```python
from build123d import *

# Parameters (mm, degrees)
SKETCH_1_R          = 20
EXTRUDE_1_DEPTH     = 200
SKETCH_2_W          = 40
SKETCH_2_H          = 40
EXTRUDE_2_DEPTH     = 50
SKETCH_3_W          = 100
SKETCH_3_H          = 30
EXTRUDE_3_DEPTH     = 40
SKETCH_4_W          = 100
SKETCH_4_H          = 30
EXTRUDE_4_DEPTH     = 40
FILLET_1_R          = 10
SKETCH_10_R         = 10
CUT_EXTRUDE_1_DEPTH = 20
EXTRUDE_6_DEPTH     = 20
EXTRUDE_7_DEPTH     = 20


with BuildPart() as part:
    # 스케치1 → 보스-돌출1 (new body)
    with BuildSketch(Plane.XY):
        Circle(SKETCH_1_R)
    extrude(amount=EXTRUDE_1_DEPTH)

    # 스케치2 → 보스-돌출2 (add)
    with BuildSketch(Plane(origin=(0, 0, 0), x_dir=(0, 0, -1), z_dir=(1, 0, 0))):
        with Locations((-20, 0)):
            Rectangle(SKETCH_2_W, SKETCH_2_H)
        with Locations((-120, 0)):
            Rectangle(SKETCH_2_W, SKETCH_2_H)
    extrude(amount=EXTRUDE_2_DEPTH)

    # 스케치3 → 보스-돌출3 (add)
    with BuildSketch(Plane(origin=(0, 0, 0), x_dir=(-1, 0, 0), z_dir=(0, 0, -1))):
        with Locations((-100, -31)):
            Rectangle(SKETCH_3_W, SKETCH_3_H)
        with Locations((-100, 31)):
            Rectangle(SKETCH_3_W, SKETCH_3_H)
    extrude(amount=-EXTRUDE_3_DEPTH)

    # 스케치4 → 보스-돌출4 (add)
    with BuildSketch(Plane(origin=(0, 0, 100), x_dir=(-1, 0, 0), z_dir=(0, 0, -1))):
        with Locations((-100, -31)):
            Rectangle(SKETCH_4_W, SKETCH_4_H)
        with Locations((-100, 31)):
            Rectangle(SKETCH_4_W, SKETCH_4_H)
    extrude(amount=-EXTRUDE_4_DEPTH)

    # 필렛1
    fillet_1_edges = [part.edges().sort_by_distance(p)[0] for p in [
        (50, -20, 20),
        (50, 20, 120),
        (50, -20, 120),
        (50, -16, 20),
        (50, 16, 20),
        (50, -16, 120),
        (50, 16, 120),
        (50, 20, 20),
    ]]
    fillet(fillet_1_edges, radius=FILLET_1_R)

    # 스케치10 → 컷-돌출1 (cut)
    with BuildSketch(Plane.XY.offset(200)):
        Circle(SKETCH_10_R)
    extrude(amount=-CUT_EXTRUDE_1_DEPTH, mode=Mode.SUBTRACT)

    # 스케치11 → 보스-돌출6 (add, symmetric)
    with BuildSketch(Plane.XY.offset(20)):
        Polygon((20, 20), (50, 38), (50, 46), (6.666666667, 20), align=None)
        Polygon((20, -20), (50, -38), (50, -46), (6.666666667, -20), align=None)
    extrude(amount=EXTRUDE_6_DEPTH, both=True)

    # 스케치13 → 보스-돌출7 (add, symmetric)
    with BuildSketch(Plane.XY.offset(120)):
        Polygon((20, 20), (50, 38), (50, 46), (6.666666667, 20), align=None)
        Polygon((20, -20), (6.666666667, -20), (50, -46), (50, -38), align=None)
    extrude(amount=EXTRUDE_7_DEPTH, both=True)


solid = part.part
```
The model under review builds one solid part; all positions refer to its coordinate system, in mm. A direction names the side the tool comes from. Coordinates: 2 decimals unless noted, no trailing zeros. Write each loop counter-clockwise with the first axis right and the second up, starting at its lowest first coordinate (ties: lowest second). Pieces come first, ordered by that corner, then holes. Notation, with made-up numbers: (7, 53.5) -> (31, 53.5) arc R24 ccw to (31, 71.5) -> close; hole circle Ø7 at (-4, 12). An arc over 180 degrees is marked (long way). One line per item, written item: value. Start each with the question number.
Q1. For faces 1 (the face through (46.99, 22.85, 19.72)), 2 (the face through (150, 31, 120)), 3 (the face through (3, -20, 120)), 4 (the face through (66, -20, 0)), 5 (the face through (50, 0, 20)), list the 3-axis set-ups (+Z, -Z, +X, -X, +Y, -Y) from which the entire face can be reached by the end or side of a thin tool; tool diameter is ignored.
Q2. Add section A-A, the plane x = 116. Give the boundary of the cut face in (y, z), then the cut area to 3 significant figures.
Q3. Clearance check with flat-ended pins moving along their axes: P1, Ø10, axis at y = 26.5, z = 60.5, coming from the -X side; P2, Ø2, axis at x = 54, y = 15.5, coming from the -Z side; P3, Ø16, axis at x = 26.5, z = 127, coming from the -Y side; P4, Ø6, axis at x = 33, z = 18.5, coming from the -Y side. State where each tip first meets the part, or that it passes through.
Q4. Add section C-C, the plane y = 0. Give the boundary of the cut face in (x, z).
Q5. To check wall thickness, follow probe 1 along Z at (x, y) = (107.5, 41); probe 2 along Y at (x, z) = (115, 125); probe 3 along Y at (x, z) = (45.5, 18). State the ranges of each line that lie inside material, in increasing order.
Q6. The part is to be moulded in two halves that separate along X. For faces 6 (the face through (3, 20, 20)), 7 (the face through (50, 34, 20)), 8 (the face through (28.637, 33.182, 119.72)), say which applies: +X half, -X half, draft (parallel to the pull), parting line (faces both ways), or undercut.
Q7. Add section D-D, the plane z = 162. Give the boundary of the cut face in (x, y), then the cut area to 3 significant figures.
Q8. Add section B-B, the plane x = 28. Give the boundary of the cut face in (y, z), then the cut area to 3 significant figures.
Response:
1. face 1: +Z, -Z
1. face 2: +Z, -Z, +X, +Y, -Y
1. face 3: +Z, -Z, -X, -Y
1. face 4: -Z, +X, -X, +Y, -Y
1. face 5: +Z, -Z, +X
2. outline: (-46, 0) -> (-16, 0) -> (-16, 40) -> (-46, 40) -> close; (-46, 100) -> (-16, 100) -> (-16, 140) -> (-46, 140) -> close; (16, 0) -> (46, 0) -> (46, 40) -> (16, 40) -> close; (16, 100) -> (46, 100) -> (46, 140) -> (16, 140) -> close
2. area: 4,800 mm²
3. P1: through
3. P2: z = 0
3. P3: y = -36.7
3. P4: y = -37.6
4. outline: (-20, 0) -> (50, 0) -> (50, 40) -> (20, 40) -> (20, 100) -> (50, 100) -> (50, 140) -> (20, 140) -> (20, 200) -> (10, 200) -> (10, 180) -> (-10, 180) -> (-10, 200) -> (-20, 200) -> close
5. probe 1: 0 to 40, 100 to 140
5. probe 2: -46 to -16, 16 to 46
5. probe 3: -43.3 to -35.3, -21.65 to 21.65, 35.3 to 43.3
6. face 6: draft
6. face 7: undercut
6. face 8: -X half
7. outline: circle Ø40 at (0, 0)
7. area: 1,260 mm²
8. outline: (-32.8, 0) -> (-24.8, 0) -> (-24.8, 40) -> (-32.8, 40) -> close; (-32.8, 100) -> (-24.8, 100) -> (-24.8, 140) -> (-32.8, 140) -> close; (-20, 0) -> (20, 0) -> (20, 40) -> (-20, 40) -> close; (-20, 100) -> (20, 100) -> (20, 140) -> (-20, 140) -> close; (24.8, 0) -> (32.8, 0) -> (32.8, 40) -> (24.8, 40) -> close; (24.8, 100) -> (32.8, 100) -> (32.8, 140) -> (24.8, 140) -> close
8. area: 4,480 mm²
